```python
from build123d import *

# Parameters (mm, degrees)
F0_W     = 133
F0_H     = 60
F1_DEPTH = 10
F2_W     = 84
F2_H     = 35.25
F3_DEPTH = 10.001
F4_SIZE  = 6
F5_R     = 5


with BuildPart() as f1:
    # F0 (on Top) → F1 (new body)
    with BuildSketch(Plane.XY):
        with Locations((-1.8318939209, -5.355308602)):
            Rectangle(F0_W, F0_H)
    extrude(amount=F1_DEPTH)

    # F2 (on face) → F3 (cut, through all)
    with BuildSketch(Plane.XY.offset(10)):
        with Locations((0.6681060791, -7.730308602)):
            Rectangle(F2_W, F2_H)
    extrude(amount=-F3_DEPTH, mode=Mode.SUBTRACT)

    # F4
    f4_edges = [f1.edges().sort_by_distance(p)[0] for p in [
        (64.668106, -5.355309, 0),
        (-68.331894, -5.355309, 0),
    ]]
    chamfer(f4_edges, length=F4_SIZE)

    # F5
    f5_edges = [f1.edges().sort_by_distance(p)[0] for p in [
        (-68.331894, -35.355309, 8),
        (-65.331894, -35.355309, 3),
        (-68.331894, 24.644691, 8),
        (-65.331894, 24.644691, 3),
        (64.668106, 24.644691, 8),
        (61.668106, 24.644691, 3),
        (64.668106, -35.355309, 8),
        (61.668106, -35.355309, 3),
    ]]
    fillet(f5_edges, radius=F5_R)


solid = f1.part
```
Geometry check sheet. Reference: the model listing, model coordinates, mm. A direction names the side the tool comes from. Coordinates: 2 decimals unless noted, no trailing zeros. Order: outer loops, then holes, each group sorted by start corner. A loop starts at its lowest first (then second) coordinate and runs counter-clockwise, first axis right, second up.
Q1. Depth check by flat-ended pin: pin 1 Ø2 at (y, z) = (-28.5, 1.5) entering from -X. Enter the tip coordinate at first touch or a pass-through.
Reply:
pin 1: stops at x = -64.83
Q2. Draft check along Y on faces 3 (the face through (42.668, -8, 5)), 4 (the face through (0, -25.355, 5)), 5 (the face through (59.96, 23.22, 3.42)), 6 (the face through (64.668, -6, 8)). Enter one of: released by +Y, released by -Y, zero draft, split by the parting line, or undercut.
Reply:
face 3: undercut
face 4: undercut
face 5: released by +Y
face 6: zero draft
Q3. Sectioned sample at B-B on y = 2. Record the cut outline in (x, z), and give its area (3 significant figures).
Reply:
outline: (-68.33, 6) - (-62.33, 0) - (-41.33, 0) - (-41.33, 10) - (-68.33, 10) - close; (42.67, 0) - (58.67, 0) - (64.67, 6) - (64.67, 10) - (42.67, 10) - close
area: 454 mm2
Q4. Tool access check on faces 1 (the face through (-41.332, -8, 5)), 2 (the face through (-65.29, -5.71, 2.96)). Record the directions out of +Z, -Z, +X, -X, +Y, -Y that give a thin tool (end or side, any length) a straight path to the whole face; none if there is none.
Reply:
face 1: +Z, -Z
face 2: -Z, -X, +Y, -Y
Q5. Thickness scan on probe 1 along X at (y, z) = (4, 6.25); probe 2 along Y at (x, z) = (33, 2); probe 3 along X at (y, z) = (1, 3.5). Record the ranges inside material, lowest first.
Reply:
probe 1: x = -68.33 to -41.33, 42.67 to 64.67
probe 2: y = -35.36 to -25.36, 9.89 to 24.64
probe 3: x = -65.83 to -41.33, 42.67 to 62.17
Q6. Sectioned sample at C-C on y = -28.5. Record the cut outline in (x, z), and give its area (3 significant figures).
Reply:
outline: (-68.33, 6) - (-62.33, 0) - (58.67, 0) - (64.67, 6) - (64.67, 10) - (-68.33, 10) - close
area: 1,290 mm2
Q7. Sectioned sample at A-A on x = -28.5. Record the cut outline in (y, z), and give its area (4 significant figures).
Reply:
outline: (-35.36, 0) - (-25.36, 0) - (-25.36, 10) - (-35.36, 10) - close; (9.89, 0) - (24.64, 0) - (24.64, 10) - (9.89, 10) - close
area: 247.5 mm2
